Could you check a few things on this drawing? It's one solid part, dimensions in mm from its lowest x, y, z. A direction names the side the tool comes from. Give positions to 0.01 mm unless a question says otherwise; leave off trailing zeros. Write each loop counter-clockwise with the first axis right and the second up, starting at its lowest first coordinate (ties: lowest second). Pieces come first, ordered by that corner, then holes. Notation, with made-up numbers: M 74,-13.75 L 97,-13.75 A16 ccw 97,-5.75 Z; hole C 85,-33 d10. An arc over 180 degrees is marked long. Answer as CSV lines item,"result". Start each with the question number.
Q1. Thinking about a two-plate mould opening in X: for the marked faces 6, 7 and 8, which applies, +X half, -X half, draft (parallel to the pull), parting line (faces both ways), or undercut?
Q2. If I drill on line 1 along Z through (x, y) = (73.5, 2.25); line 2 along Z through (x, y) = (66.5, 5) (1 decimal); line 3 along Y through (x, z) = (36.5, 14), over which ranges is the centre line in solid material (lowest first)?
Q3. Suppose I cut it at D-D (y = 11). Write out the boundary of the cut face in (x, z), then the cut area to 3 significant figures.
Q4. Suppose I cut it at C-C (y = 7.25). Write out the boundary of the cut face in (x, z), then the cut area to 3 significant figures.
Q5. Suppose I cut it at A-A (z = 39.5). Write out the boundary of the cut face in (x, y).
Q6. Suppose I cut it at B-B (x = 48). Write out the boundary of the cut face in (y, z).
Q7. On a 3-axis mill with a long thin cutter (end or side, diameter ignored), from which of +Z, -Z, +X, -X, +Y, -Y can I reach the whole of each face in a straight line? I mean the marked faces 1, 2, 3, 4 and 5. Say none if no direction works.
Q8. For pin 1 (3 mm diameter, centred on x = 31.5, y = 8, fed in from +Z); pin 2 (11 mm diameter, centred on x = 56, z = 26.5, fed in from +Y); pin 3 (1.5 mm diameter, centred on y = 11, z = 19.5, fed in from +X), each with a flat end and sliding along its axis, tell me the tip position at first contact or that it passes through.
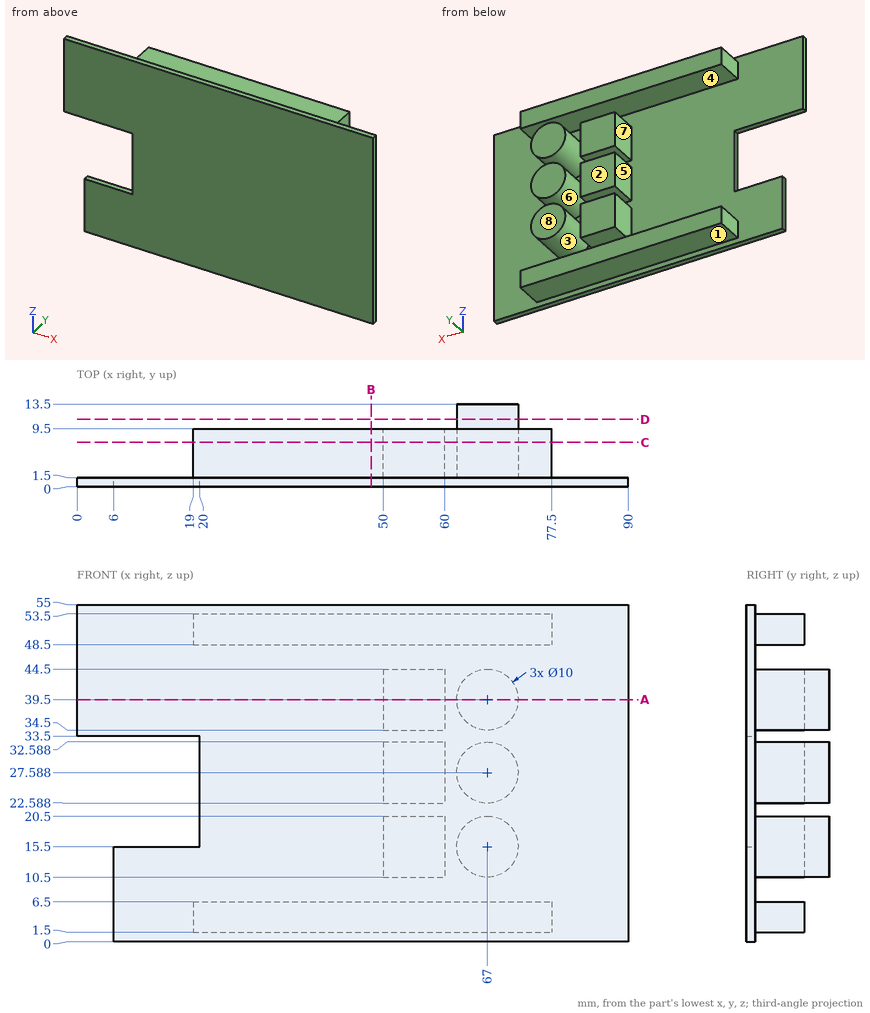
Resolved:
1,face 6,"undercut"
1,face 7,"-X half"
1,face 8,"draft"
2,line 1,"1.5 to 6.5, 48.5 to 53.5"
2,line 2,"1.5 to 6.5, 10.5 to 20.5, 22.6 to 32.6, 34.5 to 44.5, 48.5 to 53.5"
2,line 3,"0 to 1.5"
3,outline,"C 67,15.5 d10; C 67,27.59 d10; C 67,39.5 d10"
3,area,"236 mm^2"
4,outline,"M 19,1.5 L 77.5,1.5 L 77.5,6.5 L 19,6.5 Z; M 19,48.5 L 77.5,48.5 L 77.5,53.5 L 19,53.5 Z; M 50,10.5 L 60,10.5 L 60,20.5 L 50,20.5 Z; M 50,22.59 L 60,22.59 L 60,32.59 L 50,32.59 Z; M 50,34.5 L 60,34.5 L 60,44.5 L 50,44.5 Z; C 67,15.5 d10; C 67,27.59 d10; C 67,39.5 d10"
4,area,"1,120 mm^2"
5,outline,"M 0,0 L 90,0 L 90,1.5 L 72,1.5 L 72,13.5 L 62,13.5 L 62,1.5 L 60,1.5 L 60,9.5 L 50,9.5 L 50,1.5 L 0,1.5 Z"
6,outline,"M 0,0 L 1.5,0 L 1.5,1.5 L 9.5,1.5 L 9.5,6.5 L 1.5,6.5 L 1.5,48.5 L 9.5,48.5 L 9.5,53.5 L 1.5,53.5 L 1.5,55 L 0,55 Z"
7,face 1,"-Z, +X, -X, +Y"
7,face 2,"+Z, -Z, -X, +Y"
7,face 3,"+Y"
7,face 4,"+X, -X, +Y"
7,face 5,"-X, +Y"
8,pin 1,"z = 53.5"
8,pin 2,"y = 9.5"
8,pin 3,"x = 70.8"
